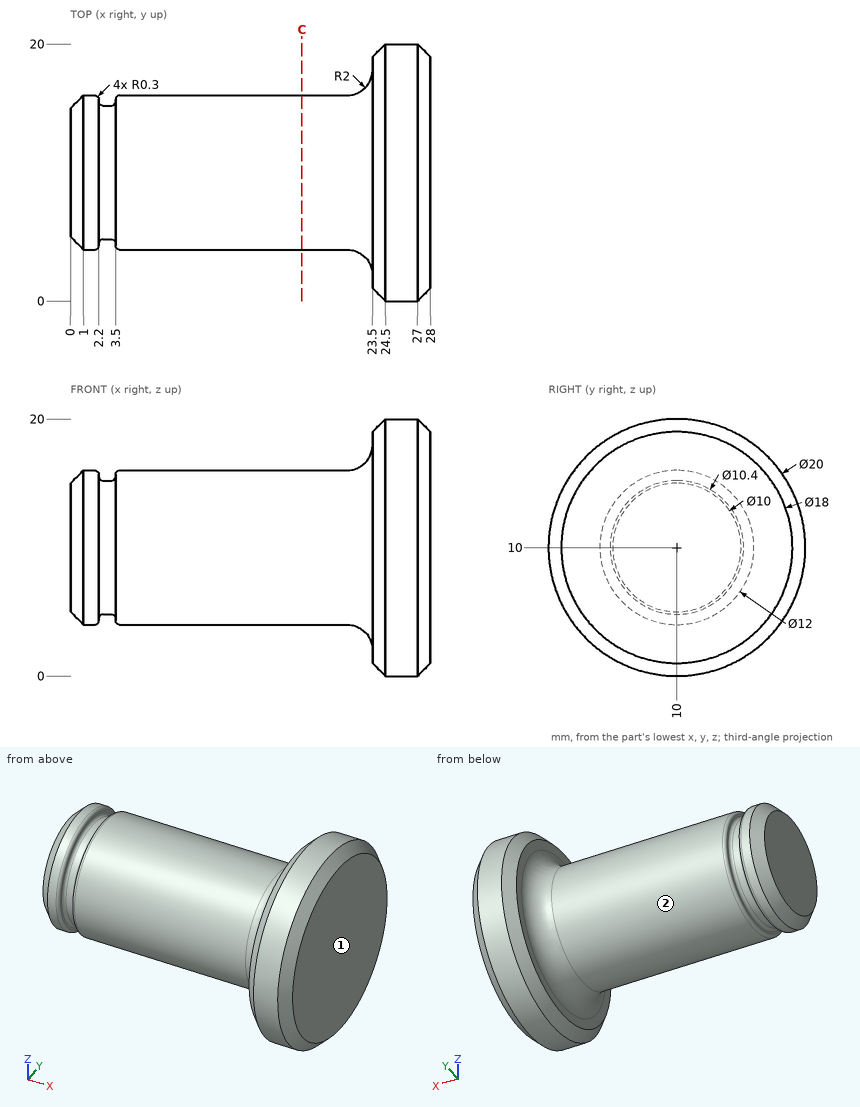
Here's the drawing with two shaded views (mm, measured from the low corner). I have some questions. A direction names the side the tool comes from. Round coordinates to 2 decimals unless told otherwise and drop trailing zeros. Order: outer loops, then holes, each group sorted by start corner. A loop starts at its lowest first (then second) coordinate and runs counter-clockwise, first axis right, second up. Notation, with made-up numbers: (66, 77.25) -> (106, 77.25) arc R17 cw to (106, 102.25) -> close; hole circle Ø11 at (26.5, 71.25). An arc over 180 degrees is marked (long way). Return JSON: item names as keys, results as strings.
Q1. For pin 1 Ø4 at (x, y) = (17, 13.5) entering from +Z; pin 2 Ø1.5 at (x, y) = (25, 4.5) entering from +Z; pin 3 Ø1 at (x, z) = (7.5, 17.5) entering from +Y; pin 4 Ø1 at (x, z) = (7.5, 12) entering from +Y, each with a flat end and sliding along its axis, tell me the tip position at first contact or that it passes through.
Filled sheet:
{"pin 1": "stops at z = 15.81", "pin 2": "stops at z = 18.8", "pin 3": "passes through", "pin 4": "stops at y = 15.81"}
Q2. Which directions (+Z, -Z, +X, -X, +Y, -Y) give clear straight access to the entire face, cutting with the end or side of a thin tool? Please do the marked faces 1 and 2.
Filled sheet:
{"face 1": "+Z, -Z, +X, +Y, -Y", "face 2": "-X"}
Q3. I need wall thicknesses on line 1 along Y through (x, z) = (15.75, 7); line 2 along X through (y, z) = (17.75, 6.5); line 3 along X through (y, z) = (15, 8). Which ranges of each line are inside material? Lowest first, please. Write a range as from..to.
Filled sheet:
{"line 1": "y = 4.8..15.2", "line 2": "x = 23.5..28", "line 3": "x = 0.39..2.22, 3.48..28"}
Q4. If we section it at C-C on x = 18: List the corners of the cut face in (y, z) for me.
Filled sheet:
{"outline": "circle Ø12 at (10, 10)"}
